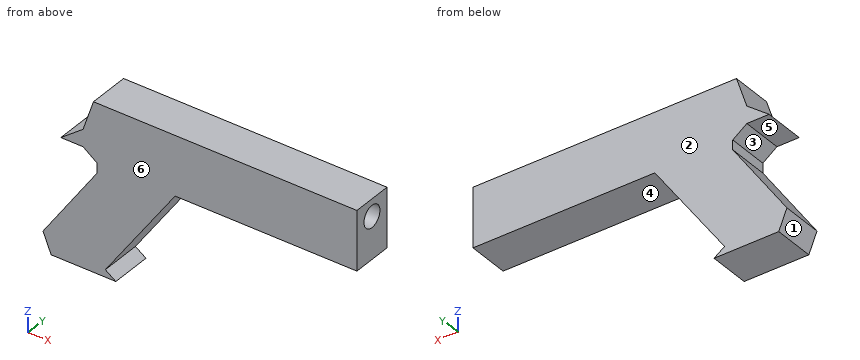
```python
from build123d import *

# Parameters (mm, degrees)
F1_DEPTH = 6.35
F2_R     = 3.37023
F3_DEPTH = 50.8


with BuildPart() as f1:
    # F0 (on Front) → F1 (new body, symmetric)
    with BuildSketch(Plane.XZ):
        Polygon((49.104851, 42.923819), (-32.16425, 42.923819), (-35.369229, 33.308882), (-42.23704, 28.043561), (-35.369229, 28.043561), (-31.019615, 24.838584), (-31.019615, 21.862533), (-47.731288, -2.403734), (-45.213088, -8.555476), (-25.255695, -8.555476), (-28.501416, -6.295493), (-6.982275, 24.609657), (49.104851, 24.609657), align=None)
    extrude(amount=F1_DEPTH, both=True)

    # F2 (on face) → F3 (cut)
    with BuildSketch(Plane.YZ.offset(49.104851)):
        with Locations((0, 37.606921)):
            Circle(F2_R)
    extrude(amount=-F3_DEPTH, mode=Mode.SUBTRACT)


solid = f1.part
```
Part model, mm, in its own coordinate system. Face numbers are marked on the shaded views. A direction names the side the tool comes from. Round coordinates to 2 decimals unless told otherwise and drop trailing zeros. Order: outer loops, then holes, each group sorted by start corner. A loop starts at its lowest first (then second) coordinate and runs counter-clockwise, first axis right, second up. Notation, with made-up numbers: M -32,31.5 L -27,31.5 A14 ccw -27,43.5 Z; hole C 7.5,35.5 d5. An arc over 180 degrees is marked long. Put each result on its own line as item: value. Start each with the question number.
1. Two-plate mould, pull along Z, no slides. Class the marked faces 1, 2 and 3: +Z half, -Z half, draft (parallel to the pull), parting line (faces both ways), or undercut.
2. Drill centre lines: probe 1 along Z at (x, y) = (19, 0); probe 2 along Z at (x, y) = (9, 4.75); probe 3 along Z at (x, y) = (-38, 5.25). Where is each one in solid material? Low to high. Write a range as [from, to].
3. Slice it at D-D on z = 12.5. List the corners of the cut face in (x, y).
4. Slice it at B-B on x = 3. List the corners of the cut face in (y, z).
5. Slice it at C-C on z = 18. List the corners of the cut face in (x, y).
6. Tool access for the marked faces 4, 5 and 6: list every direction of +Z, -Z, +X, -X, +Y, -Y with a clear straight run to the whole face (end or side of a thin tool).
7. Slice it at A-A on y = 0. List the corners of the cut face in (x, z).
8. Drop flat-ended pins along their axis: pin 1 (3 mm diameter, centred on y = 3, z = 37, fed in from -X); pin 2 (1 mm diameter, centred on y = 1.5, z = 8.5, fed in from -X); pin 3 (1.5 mm diameter, centred on y = 2.5, z = 23.5, fed in from -X). Give the stop position or say it passes through.
Findings:
1. face 1: -Z half
1. face 2: draft
1. face 3: undercut
2. probe 1: [24.61, 34.24], [40.98, 42.92]
2. probe 2: [24.61, 42.92]
2. probe 3: [-8.56, 11.73], [28.04, 31.29]
3. outline: M -37.47,-6.35 L -15.41,-6.35 L -15.41,6.35 L -37.47,6.35 Z
4. outline: M -6.35,24.61 L 6.35,24.61 L 6.35,42.92 L -6.35,42.92 Z; hole C 0,37.61 d6.74
5. outline: M -33.68,-6.35 L -11.58,-6.35 L -11.58,6.35 L -33.68,6.35 Z
6. face 4: -Z, +X, +Y, -Y
6. face 5: -X, +Y, -Y
6. face 6: +Z, -Z, +X, -X, -Y
7. outline: M -47.73,-2.4 L -45.21,-8.56 L -25.26,-8.56 L -28.5,-6.3 L -6.98,24.61 L 49.1,24.61 L 49.1,34.24 L -1.7,34.24 L -1.7,40.98 L 49.1,40.98 L 49.1,42.92 L -32.16,42.92 L -35.37,33.31 L -42.24,28.04 L -35.37,28.04 L -31.02,24.84 L -31.02,21.86 Z
8. pin 1: x = -34.64
8. pin 2: x = -40.57
8. pin 3: x = -31.02
